from build123d import *

# Parameters (mm, degrees)
F0_R     = 2.5
F1_DEPTH = 8.89
F0_R_2   = 4.786
F2_DEPTH = 3.81
F0_R_3   = 11
F3_DEPTH = 2.54
F4_R     = 1.5
F5_DEPTH = 7.62


with BuildPart() as f1:
    # F0 (on Top) → F1 (new body)
    with BuildSketch(Plane.XY):
        Circle(F0_R)
    extrude(amount=F1_DEPTH)

    # F0 (on Top) → F2 (join)
    with BuildSketch(Plane.XY):
        Circle(F0_R_2)
        Circle(F0_R, mode=Mode.SUBTRACT)
    extrude(amount=F2_DEPTH)

    # F0 (on Top) → F3 (join)
    with BuildSketch(Plane.XY):
        Circle(F0_R_3)
        Circle(F0_R_2, mode=Mode.SUBTRACT)
    extrude(amount=F3_DEPTH)

    # F4 (on face) → F5 (cut)
    with BuildSketch(Plane.XY.offset(8.89)):
        Circle(F4_R)
    extrude(amount=-F5_DEPTH, mode=Mode.SUBTRACT)


solid = f1.part
Model file for the job. Use its own axes, mm. A direction names the side the tool comes from. Round coordinates to 2 decimals unless told otherwise and drop trailing zeros. Order: outer loops, then holes, each group sorted by start corner. A loop starts at its lowest first (then second) coordinate and runs counter-clockwise, first axis right, second up.
(1) 3-axis set-ups, long thin cutter, end or side, ignore diameter. For faces 1 (the face through (-2.38, -10.74, 1.25)), 2 (the face through (2, -5, 2.54)): which of +Z, -Z, +X, -X, +Y, -Y reach the whole face in a straight line?
(2) Pin check, flat tips, straight feed: pin 1 (3 mm diameter, centred on y = -2.5, z = 5.5, fed in from +X); pin 2 (2 mm diameter, centred on x = 6.5, y = -3, fed in from +Z); pin 3 (4 mm diameter, centred on x = 1.5, z = 5.5, fed in from -Y). Stop position of each tip, or through.
(3) Band-saw the part on C-C (z = 3.5). List the corners of the cut face in (x, y).
(4) Band-saw the part on D-D (x = -4.25). List the corners of the cut face in (y, z).
(5) Drill centre lines: line 1 (Y direction, x = 0, z = 6.5); line 2 (Z direction, x = 2.25, y = 9.5); line 3 (Y direction, x = 0, z = 3.25). Where is each one in solid material? Low to high.
(6) Band-saw the part on A-A (x = 0). List the corners of the cut face in (y, z).
(7) Pull direction X, two halves, no side cores. Call faces 3 (the face through (2, -2, 3.81)), 4 (the face through (0, 0, 1.27)), 5 (the face through (4.565, 1.438, 3.166)): released by +X, released by -X, zero draft, split by the parting line, or undercut.
Verdict:
1. face 1: +Z, -Z
1. face 2: +Z
2. pin 1: stops at x = 2.29
2. pin 2: stops at z = 2.54
2. pin 3: stops at y = -4.77
3. outline: circle Ø9.57 at (0, 0); hole circle Ø3 at (0, 0)
4. outline: (-10.15, 0) - (10.15, 0) - (10.15, 2.54) - (2.2, 2.54) - (2.2, 3.81) - (-2.2, 3.81) - (-2.2, 2.54) - (-10.15, 2.54) - close
5. line 1: y = -2.5 to -1.5, 1.5 to 2.5
5. line 2: z = 0 to 2.54
5. line 3: y = -4.79 to -1.5, 1.5 to 4.79
6. outline: (-11, 0) - (11, 0) - (11, 2.54) - (4.79, 2.54) - (4.79, 3.81) - (2.5, 3.81) - (2.5, 8.89) - (1.5, 8.89) - (1.5, 1.27) - (-1.5, 1.27) - (-1.5, 8.89) - (-2.5, 8.89) - (-2.5, 3.81) - (-4.79, 3.81) - (-4.79, 2.54) - (-11, 2.54) - close
7. face 3: zero draft
7. face 4: undercut
7. face 5: split by the parting line
